The listing builds one solid part. Answer for the finished solid, in the listing's coordinates (mm). Give positions to 0.01 mm unless a question says otherwise; leave off trailing zeros. Loops run counter-clockwise (first coordinate to the right, second up) from the corner with the lowest first, then second, coordinate; pieces in that order, holes last. Notation, with made-up numbers: M -35.75,76 L 18.25,76 A25 cw 18.25,92 Z; hole C 35,3.25 d4. An arc over 180 degrees is marked long. One line per item, written item: value. Start each with the question number.
Q1. A flat-ended cylindrical pin translates along its axis: pin 1 (8.5 mm diameter, centred on x = 151.2, z = 65.405, fed in from -Y) (3 decimals). Find the tip coordinate at first contact, or state that the pin passes through.
Q2. A cutting plane is placed at D-D, the plane y = 0.25. State how many separate pieces and enclosed holes the cut face has, and give its area (3 significant figures).
Q3. A cutting plane is placed at C-C, the plane z = 30.48. Determine the outline of the cut face in (x, y) (3 decimals), and give its area (3 significant figures).
Q4. A cutting plane is placed at B-B, the plane z = 0. Determine the outline of the cut face in (x, y) (3 decimals), and give its area (3 significant figures).
Q5. A cutting plane is placed at A-A, the plane x = 30.48. Determine the outline of the cut face in (y, z) (3 decimals), and give its area (3 significant figures).
Q6. The mould has two halves that part along X. Classify faces 1 (the flat face through (-3, 3.175, 30)), 2 (the cylindrical face through (31.86, -0.04, -24.28)): +X half, -X half, draft (parallel to the pull), parting line (faces both ways), or undercut.
Q7. Consider L1, parallel to Z at x = -151.2, y = 0.25; L2, parallel to X at y = -1.5, z = 30.48; L3, parallel to Z at x = 30.48, y = 1.5. Determine where each line is inside the solid, lowest interval first.
from build123d import *

# Parameters (mm, degrees)
SKETCH1_W                   = 457.2
SKETCH1_H                   = 116.84
BOSS_EXTRUDE1_DEPTH         = 3.175
F_1_1_DIAMETER_HOLE1_D      = 50.8
F_1_2_0_5_DIAMETER_HOLE1_D  = 12.7
F_4_0_4_DIAMETER_HOLE1_D    = 4.2164
F_1_4_0_25_DIAMETER_HOLE1_D = 6.35
AUX_CLEARANCE_HOLES_REACH   = 8.35
SKETCH11_R                  = 3.175


with BuildPart() as part:
    # Sketch1 → Boss-Extrude1 (new body, symmetric)
    with BuildSketch(Plane(origin=(0, 0, 0), x_dir=(1, 0, 0), z_dir=(0, 1, 0))):
        with Locations((0, -17.78)):
            Rectangle(SKETCH1_W, SKETCH1_H)
    extrude(amount=BOSS_EXTRUDE1_DEPTH, both=True)

    # 1 (1) Diameter Hole1 (through all)
    with Locations(Plane(origin=(0, 3.175, 0), x_dir=(1, 0, 0), z_dir=(0, 1, 0))):
        with Locations((0, 0)):
            Hole(F_1_1_DIAMETER_HOLE1_D / 2)

    # 1/2 (0.5) Diameter Hole1 (through all)
    with Locations(Plane(origin=(0, 3.175, 0), x_dir=(1, 0, 0), z_dir=(0, 1, 0))):
        with Locations((30.48, -30.48), (-30.48, 30.48), (-30.48, -30.48), (30.48, 30.48)):
            Hole(F_1_2_0_5_DIAMETER_HOLE1_D / 2)

    # Ø4.0 (4) Diameter Hole1 (through all)
    with Locations(Plane(origin=(0, 3.175, 0), x_dir=(1, 0, 0), z_dir=(0, 1, 0))):
        with Locations((0, -55.63), (0, -69.63)):
            Hole(F_4_0_4_DIAMETER_HOLE1_D / 2)

    # 1/4 (0.25) Diameter Hole1 (through all)
    with Locations(Plane(origin=(0, 3.175, 0), x_dir=(1, 0, 0), z_dir=(0, 1, 0))):
        with Locations((75, -65.405), (-75, 29.845), (-75, -65.405), (75, 29.845)):
            Hole(F_1_4_0_25_DIAMETER_HOLE1_D / 2)

    # Sketch11 → Aux Clearance holes (cut, up to next)
    with BuildSketch(Plane(origin=(0, 3.175, 0), x_dir=(1, 0, 0), z_dir=(0, 1, 0)), mode=Mode.PRIVATE) as aux_clearance_holes_sk1:
        with Locations((-151.2, 29.845)):
            Circle(SKETCH11_R)
    aux_clearance_holes_tool1 = extrude(aux_clearance_holes_sk1.sketch, amount=-AUX_CLEARANCE_HOLES_REACH, mode=Mode.PRIVATE) & part.part
    add(aux_clearance_holes_tool1.solids().sort_by_distance((-151.2, 3.175, -29.845))[0], mode=Mode.SUBTRACT)
    # Sketch11 → Aux Clearance holes (cut, up to next)
    with BuildSketch(Plane(origin=(0, 3.175, 0), x_dir=(1, 0, 0), z_dir=(0, 1, 0)), mode=Mode.PRIVATE) as aux_clearance_holes_sk2:
        with Locations((-151.2, -65.405)):
            Circle(SKETCH11_R)
    aux_clearance_holes_tool2 = extrude(aux_clearance_holes_sk2.sketch, amount=-AUX_CLEARANCE_HOLES_REACH, mode=Mode.PRIVATE) & part.part
    add(aux_clearance_holes_tool2.solids().sort_by_distance((-151.2, 3.175, 65.405))[0], mode=Mode.SUBTRACT)
    # Sketch11 → Aux Clearance holes (cut, up to next)
    with BuildSketch(Plane(origin=(0, 3.175, 0), x_dir=(1, 0, 0), z_dir=(0, 1, 0)), mode=Mode.PRIVATE) as aux_clearance_holes_sk3:
        with Locations((151.2, 29.845)):
            Circle(SKETCH11_R)
    aux_clearance_holes_tool3 = extrude(aux_clearance_holes_sk3.sketch, amount=-AUX_CLEARANCE_HOLES_REACH, mode=Mode.PRIVATE) & part.part
    add(aux_clearance_holes_tool3.solids().sort_by_distance((151.2, 3.175, -29.845))[0], mode=Mode.SUBTRACT)
    # Sketch11 → Aux Clearance holes (cut, up to next)
    with BuildSketch(Plane(origin=(0, 3.175, 0), x_dir=(1, 0, 0), z_dir=(0, 1, 0)), mode=Mode.PRIVATE) as aux_clearance_holes_sk4:
        with Locations((151.2, -65.405)):
            Circle(SKETCH11_R)
    aux_clearance_holes_tool4 = extrude(aux_clearance_holes_sk4.sketch, amount=-AUX_CLEARANCE_HOLES_REACH, mode=Mode.PRIVATE) & part.part
    add(aux_clearance_holes_tool4.solids().sort_by_distance((151.2, 3.175, 65.405))[0], mode=Mode.SUBTRACT)


solid = part.part
Answer block:
1. pin 1: y = -3.175
2. separate pieces: 1
2. enclosed holes: 15
2. area: 50,600 mm^2
3. outline: M -228.6,-3.175 L -36.83,-3.175 L -36.83,3.175 L -228.6,3.175 Z; M -24.13,-3.175 L 24.13,-3.175 L 24.13,3.175 L -24.13,3.175 Z; M 36.83,-3.175 L 228.6,-3.175 L 228.6,3.175 L 36.83,3.175 Z
3. area: 2,740 mm^2
4. outline: M -228.6,-3.175 L -25.4,-3.175 L -25.4,3.175 L -228.6,3.175 Z; M 25.4,-3.175 L 228.6,-3.175 L 228.6,3.175 L 25.4,3.175 Z
4. area: 2,580 mm^2
5. outline: M -3.175,-40.64 L 3.175,-40.64 L 3.175,-36.83 L -3.175,-36.83 Z; M -3.175,-24.13 L 3.175,-24.13 L 3.175,24.13 L -3.175,24.13 Z; M -3.175,36.83 L 3.175,36.83 L 3.175,76.2 L -3.175,76.2 Z
5. area: 581 mm^2
6. face 1: draft
6. face 2: undercut
7. L1: -40.64 to -33.02, -26.67 to 62.23, 68.58 to 76.2
7. L2: -228.6 to -36.83, -24.13 to 24.13, 36.83 to 228.6
7. L3: -40.64 to -36.83, -24.13 to 24.13, 36.83 to 76.2
